Model file for the job. Use its own axes, mm. Face numbers are marked on the shaded views. A direction names the side the tool comes from. Coordinates: 2 decimals unless noted, no trailing zeros. Loops run counter-clockwise (first coordinate to the right, second up) from the corner with the lowest first, then second, coordinate; pieces in that order, holes last. Notation, with made-up numbers: M 59,16 L 79,16 A29 ccw 79,49 Z; hole C -18.75,68.25 d11. An arc over 180 degrees is marked long. Write item = value, one per line. Start each with the question number.
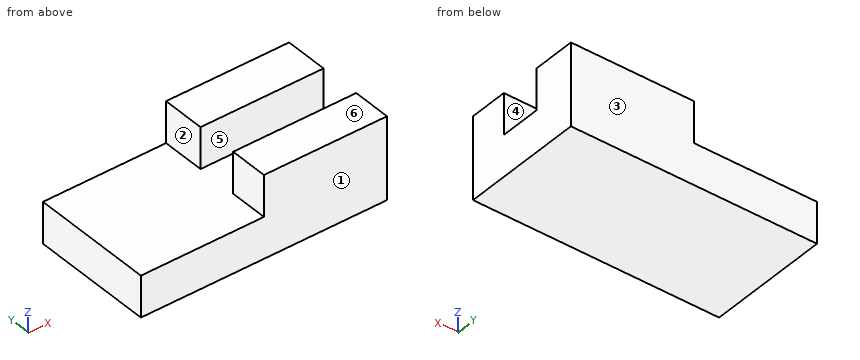
from build123d import *

# Parameters (mm, degrees)
F0_W     = 152.4
F0_H     = 50.8
F1_DEPTH = 76.2
F2_W     = 76.2
F2_H     = 25.4
F3_DEPTH = 25.4
F5_DEPTH = 25.4


with BuildPart() as f1:
    # F0 (on Front) → F1 (new body)
    with BuildSketch(Plane.XZ):
        with Locations((76.2, 25.4)):
            Rectangle(F0_W, F0_H)
    extrude(amount=F1_DEPTH)

    # F2 (on face) → F3 (cut)
    with BuildSketch(Plane.XY.offset(50.8)):
        with Locations((114.3, -39.528749)):
            Rectangle(F2_W, F2_H)
    extrude(amount=-F3_DEPTH, mode=Mode.SUBTRACT)

    # F4 (on face) → F5 (cut)
    with BuildSketch(Plane.XY.offset(50.8)):
        Polygon((76.2, -26.828749), (76.2, 0), (0, 0), (0, -76.2), (76.2, -76.2), (76.2, -52.228749), align=None)
    extrude(amount=-F5_DEPTH, mode=Mode.SUBTRACT)


solid = f1.part
Item 1: Pull direction Y, two halves, no side cores. Call the marked faces 3, 4, 5 and 6: +Y half, -Y half, draft (parallel to the pull), parting line (faces both ways), or undercut.
Item 2: Pin check, flat tips, straight feed: pin 1 Ø3 at (y, z) = (-30, 41) entering from +X; pin 2 Ø19 at (y, z) = (-62, 35.5) entering from -X; pin 3 Ø3 at (x, y) = (68.5, -51) entering from +Z. Stop position of each tip, or through.
Item 3: Probe L1, parallel to Y at x = 131, z = 49; L2, parallel to Z at x = 36.5, y = -62; L3, parallel to X at y = -22, z = 36.5. List the from-to ranges inside material, lowest first.
Item 4: 3-axis set-ups, long thin cutter, end or side, ignore diameter. For the marked faces 1 and 2: which of +Z, -Z, +X, -X, +Y, -Y reach the whole face in a straight line?
Item 5: Cut at A-A (z = 28). Give the cut face in (x, y).
Item 6: Cut at B-B (x = 93). Give the cut face in (y, z).
Item 7: Cut at D-D (x = 41). Give the cut face in (y, z), plus the area to 3 significant figures.
Item 8: Cut at C-C (y = -16). Give the cut face in (x, z), plus the area to 3 significant figures.
Reported:
q1.face_3 = +Y half
q1.face_4 = undercut
q1.face_5 = undercut
q1.face_6 = draft
q2.pin_1 = through
q2.pin_2 = 76.2
q2.pin_3 = 25.4
q3.L1 = -76.2 to -52.23, -26.83 to 0
q3.L2 = 0 to 25.4
q3.L3 = 76.2 to 152.4
q4.face_1 = +Z, -Z, +X, -X, -Y
q4.face_2 = +Z, -X, +Y, -Y
q5.outline = M 76.2,-76.2 L 152.4,-76.2 L 152.4,-52.23 L 76.2,-52.23 Z; M 76.2,-26.83 L 152.4,-26.83 L 152.4,0 L 76.2,0 Z
q6.outline = M -76.2,0 L 0,0 L 0,50.8 L -26.83,50.8 L -26.83,25.4 L -52.23,25.4 L -52.23,50.8 L -76.2,50.8 Z
q7.outline = M -76.2,0 L 0,0 L 0,25.4 L -76.2,25.4 Z
q7.area = 1,940 mm^2
q8.outline = M 0,0 L 152.4,0 L 152.4,50.8 L 76.2,50.8 L 76.2,25.4 L 0,25.4 Z
q8.area = 5,810 mm^2
